Input: dimensioned drawing with shaded views. Units: mm. Origin: part minimum x, y, z. Give positions to 0.01 mm unless a question says otherwise; leave off trailing zeros. Write each loop counter-clockwise with the first axis right and the second up, starting at its lowest first coordinate (ties: lowest second). Pieces come first, ordered by that corner, then holes.
Q1. Section A-A (x = 12). Return the cut outline in (y, z).
Q2. Line query: line 1 (Z direction, x = 16, y = 26.5); line 2 (Z direction, x = 13.5, y = 24); line 3 (X direction, y = 16, z = 1.25). Output: solid intervals per line, ascending.
Q3. Pin query (flat end, axial travel): pin 1 Ø2 at (x, y) = (16, 6.5) entering from -Z; pin 2 Ø3 at (x, z) = (13.925, 13.925) entering from -Y. Return the tip coordinate at first contact, or that it passes through.
Q4. Section B-B (y = 27.5). Return the cut outline in (x, z) (3 decimals), plus the area to 3 significant figures.
Q5. Section C-C (z = 15.25). Return the cut outline in (x, y) (3 decimals).
Q6. Mould query, pull axis X, two halves, no side actions, for the marked faces 1, 2 and 3. Classes: +X half, -X half, draft (parallel to the pull), parting line (faces both ways), or undercut.
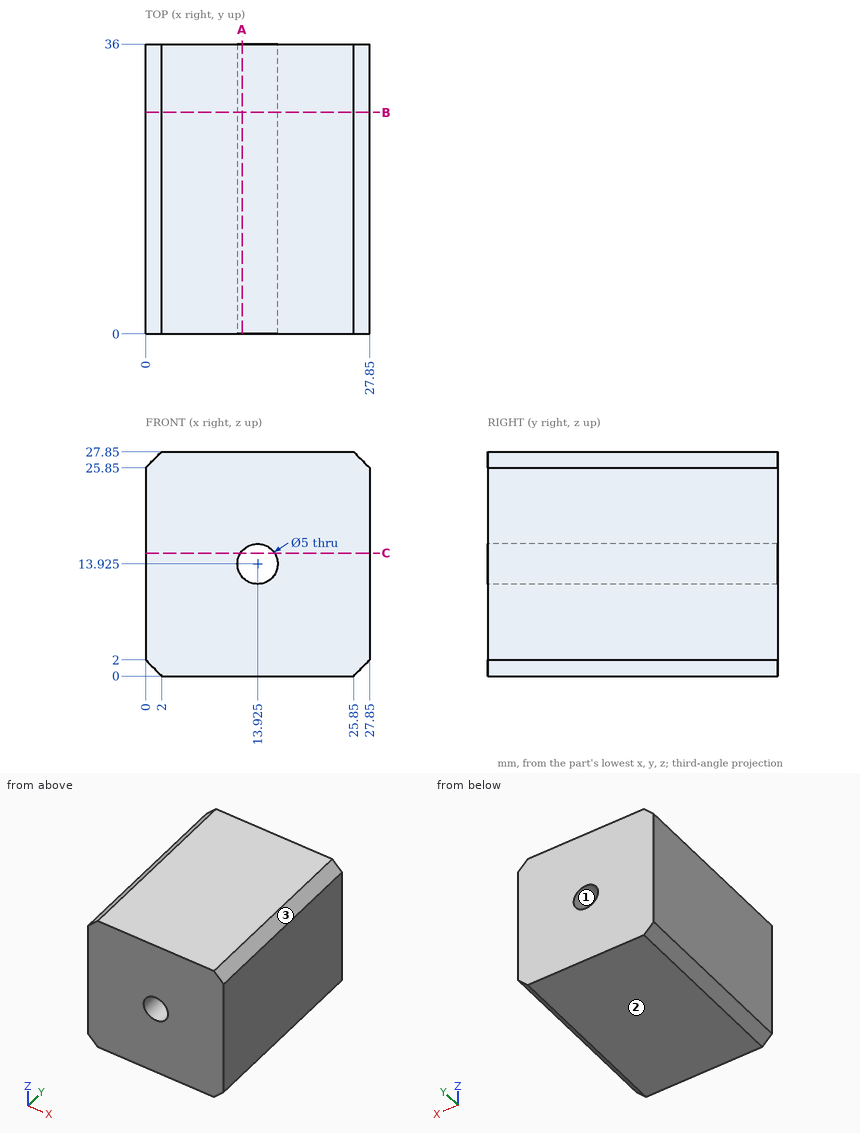
Computed:
1. outline: (0, 0) - (36, 0) - (36, 12.33) - (0, 12.33) - close; (0, 15.52) - (36, 15.52) - (36, 27.85) - (0, 27.85) - close
2. line 1: z = 0 to 12.53, 15.32 to 27.85
2. line 2: z = 0 to 11.46, 16.39 to 27.85
2. line 3: x = 0.75 to 27.1
3. pin 1: stops at z = 0
3. pin 2: passes through
4. outline: (0, 2) - (2, 0) - (25.85, 0) - (27.85, 2) - (27.85, 25.85) - (25.85, 27.85) - (2, 27.85) - (0, 25.85) - close; hole circle Ø5 at (13.925, 13.925)
4. area: 748 mm2
5. outline: (0, 0) - (11.805, 0) - (11.805, 36) - (0, 36) - close; (16.045, 0) - (27.85, 0) - (27.85, 36) - (16.045, 36) - close
6. face 1: undercut
6. face 2: draft
6. face 3: +X half
